from build123d import *

# Parameters (mm, degrees)
SKETCH1_R                                           = 50
BOSS_EXTRUDE1_DEPTH                                 = 2.5
CBORE_FOR_00_BINDING_HEAD_MACHINE_SCREW_D           = 1.397
CBORE_FOR_00_BINDING_HEAD_MACHINE_SCREW_DEPTH       = 7.5
CBORE_FOR_00_BINDING_HEAD_MACHINE_SCREW_CBORE_D     = 3.175
CBORE_FOR_00_BINDING_HEAD_MACHINE_SCREW_CBORE_DEPTH = 0.7112
CBORE_FOR_00_BINDING_HEAD_MACHINE_SCREW_TIP         = 0.419701142


with BuildPart() as part:
    # Sketch1 → Boss-Extrude1 (new body)
    with BuildSketch(Plane(origin=(0, 0, 0), x_dir=(1, 0, 0), z_dir=(0, 1, 0))):
        with Locations(Location((0, 0, 0), (0, 0, 270))):
            Circle(SKETCH1_R)
    extrude(amount=BOSS_EXTRUDE1_DEPTH)

    # CBORE for #00 Binding Head Machine Screw1
    with Locations(Plane(origin=(-15.891003533, 0, -43.270503311), x_dir=(0, 0, -1), z_dir=(0, -1, 0))):
        with Locations((0, 0), (-59.161506844, -27.379499778), (-86.541006622, 31.782007066), (-27.379499778, 59.161506844)):
            CounterBoreHole(CBORE_FOR_00_BINDING_HEAD_MACHINE_SCREW_D / 2, CBORE_FOR_00_BINDING_HEAD_MACHINE_SCREW_CBORE_D / 2, CBORE_FOR_00_BINDING_HEAD_MACHINE_SCREW_CBORE_DEPTH, depth=CBORE_FOR_00_BINDING_HEAD_MACHINE_SCREW_DEPTH)
            with Locations((0, 0, -(CBORE_FOR_00_BINDING_HEAD_MACHINE_SCREW_DEPTH + CBORE_FOR_00_BINDING_HEAD_MACHINE_SCREW_TIP / 2))):  # 118° drill point
                Cone(0, CBORE_FOR_00_BINDING_HEAD_MACHINE_SCREW_D / 2, CBORE_FOR_00_BINDING_HEAD_MACHINE_SCREW_TIP, mode=Mode.SUBTRACT)


solid = part.part
Design review of the part built by this model. Coordinates are the model's own, in mm. A direction names the side the tool comes from. Round coordinates to 2 decimals unless told otherwise and drop trailing zeros. Write each loop counter-clockwise with the first axis right and the second up, starting at its lowest first coordinate (ties: lowest second). Pieces come first, ordered by that corner, then holes.
Item 1: Consider section B-B on z = 31. Give the boundary of the cut face in (x, y).
Item 2: Wall thickness on L1, parallel to X at y = 1.2, z = -1; L2, parallel to Z at x = -9, y = 1.4; L3, parallel to X at y = 1.75, z = 31.5: over which ranges is each line inside the solid? List them lowest first.
Item 3: For faces 1 (the cylindrical face through (-17.44, 0.35, -42.93)), 2 (the flat face through (1, 0, -1)), list the 3-axis set-ups (+Z, -Z, +X, -X, +Y, -Y) from which the entire face can be reached by the end or side of a thin tool; tool diameter is ignored.
Item 4: Consider section A-A on y = 1.1. Give the boundary of the cut face in (x, z).
Item 5: Draft analysis for pull direction Z (two halves, no side actions). For faces 3 (the flat face through (1, 2.5, -1)), 4 (the flat face through (43, 0.711, -17)), 5 (the cylindrical face through (15.02, 1.23, 47.69)), state which applies: released by +Z, released by -Z, zero draft, split by the parting line, or undercut.
Item 6: Consider section C-C on x = -30.5. Give the boundary of the cut face in (y, z), and give its area (3 significant figures).
Item 7: For pin 1 Ø1.5 at (y, z) = (1.5, 33) entering from +X; pin 2 Ø1.9 at (x, z) = (43.27, -15.89) entering from -Y; pin 3 Ø1.5 at (x, y) = (3, 0.5) entering from -Z, all flat-tipped, find the tip position at first contact; note any pin that passes through.
Check values:
1. outline: (-39.23, 0) - (39.23, 0) - (39.23, 2.5) - (-39.23, 2.5) - close
2. L1: x = -49.99 to 49.99
2. L2: z = -49.18 to 49.18
2. L3: x = -38.83 to 38.83
3. face 1: -Y
3. face 2: +Z, -Z, +X, -X, -Y
4. outline: circle Ø100 at (0, 0); hole circle Ø1.4 at (-43.27, 15.89); hole circle Ø1.4 at (-15.89, -43.27); hole circle Ø1.4 at (15.89, 43.27); hole circle Ø1.4 at (43.27, -15.89)
5. face 3: zero draft
5. face 4: undercut
5. face 5: split by the parting line
6. outline: (0, -39.62) - (2.5, -39.62) - (2.5, 39.62) - (0, 39.62) - close
6. area: 198 mm2
7. pin 1: stops at x = 38.21
7. pin 2: stops at y = 0.71
7. pin 3: stops at z = -49.95
